Geometry: final body of the model. Coordinates: model frame, mm. Face numbers are marked on the shaded views. A direction names the side the tool comes from. Give positions to 0.01 mm unless a question says otherwise; leave off trailing zeros. Write each loop counter-clockwise with the first axis right and the second up, starting at its lowest first coordinate (ties: lowest second). Pieces come first, ordered by that corner, then holes.
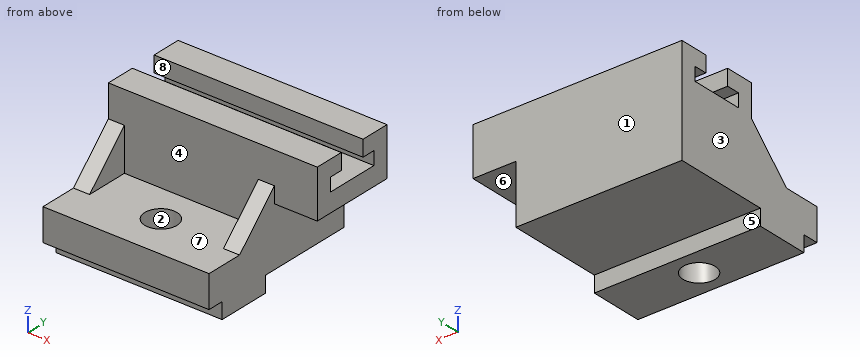
from build123d import *

# Parameters (mm, degrees)
F0_W      = 98.425
F0_H      = 19.05
F1_DEPTH  = 98.425
F2_W      = 98.425
F2_H      = 31.75
F3_DEPTH  = 9.525
F5_DEPTH  = 58.928
F6_W      = 98.425
F6_H      = 50.8
F7_DEPTH  = 44.45
F8_W      = 98.425
F8_H      = 15.875
F9_DEPTH  = 17.4625
F10_W     = 7.9375
F10_H     = 7.9375
F11_DEPTH = 104.394
F13_DEPTH = 25.4
F14_W     = 9.525
F14_H     = 25.4
F15_DEPTH = 31.242
F17_DEPTH = 25.4
F19_DEPTH = 39.878
F21_DEPTH = 25.4


with BuildPart() as f1:
    # F0 (on Front) → F1 (new body)
    with BuildSketch(Plane.XZ):
        with Locations((16.241223073, -7.6058536083)):
            Rectangle(F0_W, F0_H)
    extrude(amount=F1_DEPTH)

    # F2 (on face) → F3 (join)
    with BuildSketch(Plane(origin=(0, 0, -17.1308536083), x_dir=(1, 0, 0), z_dir=(0, 0, -1))):
        with Locations((16.241223073, 73.025)):
            Rectangle(F2_W, F2_H)
    extrude(amount=F3_DEPTH)

    # F4 (on face) → F5 (cut)
    with BuildSketch(Plane.XY.offset(1.9191463917)):
        with BuildLine():
            ThreePointArc((16.241223073, -82.55), (22.9764151638, -79.7601920908), (25.766223073, -73.025))
            ThreePointArc((25.766223073, -73.025), (9.5060309822, -66.2898079092), (16.241223073, -82.55))
        make_face()
    extrude(amount=-F5_DEPTH, mode=Mode.SUBTRACT)

    # F6 (on face) → F7 (join)
    with BuildSketch(Plane.XY.offset(1.9191463917)):
        with Locations((16.241223073, -25.4)):
            Rectangle(F6_W, F6_H)
    extrude(amount=F7_DEPTH)

    # F8 (on face) → F9 (cut)
    with BuildSketch(Plane.XY.offset(46.3691463917)):
        with Locations((16.241223073, -25.4)):
            Rectangle(F8_W, F8_H)
    extrude(amount=-F9_DEPTH, mode=Mode.SUBTRACT)

    # F10 (on face) → F11 (cut)
    with BuildSketch(Plane(origin=(-32.971276927, 0, 0), x_dir=(0, -1, 0), z_dir=(-1, 0, 0))):
        with Locations((13.49375, 32.8753963917)):
            Rectangle(F10_W, F10_H)
        with Locations((37.30625, 32.8753963917)):
            Rectangle(F10_W, F10_H)
    extrude(amount=-F11_DEPTH, mode=Mode.SUBTRACT)

    # F12 (on face) → F13 (join)
    with BuildSketch(Plane.YZ.offset(65.453723073)):
        Polygon((-33.3375, 46.3691463917), (-50.8, 46.3691463917), (-50.8, 17.7941463917), (0, 17.7941463917), (0, 46.3691463917), (-17.4625, 46.3691463917), (-17.4625, 36.8441463917), (-9.525, 36.8441463917), (-9.525, 28.9066463917), (-41.275, 28.9066463917), (-41.275, 36.8441463917), (-33.3375, 36.8441463917), align=None)
    extrude(amount=F13_DEPTH)

    # F14 (on face) → F15 (join)
    with BuildSketch(Plane.XZ.offset(50.8)):
        with Locations((-28.208776927, 14.6191463917)):
            Rectangle(F14_W, F14_H)
    extrude(amount=F15_DEPTH)

    # F16 (on face) → F17 (cut)
    with BuildSketch(Plane.YZ.offset(-23.446276927)):
        Polygon((-76.2, 1.9191463917), (-50.8, 27.3191463917), (-82.042, 27.3191463917), (-82.042, 1.9191463917), align=None)
    extrude(amount=-F17_DEPTH, mode=Mode.SUBTRACT)

    # F18 (on face) → F19 (join)
    with BuildSketch(Plane.XZ.offset(50.8)):
        Polygon((55.928723073, 1.9191463917), (65.453723073, 1.9191463917), (65.453723073, 17.7941463917), (65.453723073, 27.3191463917), (55.928723073, 27.3191463917), align=None)
    extrude(amount=F19_DEPTH)

    # F20 (on face) → F21 (cut)
    with BuildSketch(Plane(origin=(55.928723073, 0, 0), x_dir=(0, -1, 0), z_dir=(-1, 0, 0))):
        Polygon((90.678, 27.3191463917), (50.8, 27.3191463917), (76.2, 1.9191463917), (90.678, 1.9191463917), align=None)
    extrude(amount=-F21_DEPTH, mode=Mode.SUBTRACT)


solid = f1.part
Q1. Section D-D on y = -43.5. Output: boundary loops of the cut face in (x, z), plus the area to 3 significant figures.
Filled sheet:
outline: (-32.97, -17.13) - (65.45, -17.13) - (65.45, 17.79) - (90.85, 17.79) - (90.85, 46.37) - (-32.97, 46.37) - close
area: 6,980 mm2
Q2. Pull-direction query (X, two-part tool) for the marked faces 1, 2, 3 and 4; classes: released by +X, released by -X, zero draft, split by the parting line, or undercut.
Filled sheet:
face 1: zero draft
face 2: undercut
face 3: released by -X
face 4: undercut
Q3. Section C-C on y = -80.5. Output: boundary loops of the cut face in (x, z), plus the area to 3 significant figures.
Filled sheet:
outline: (-32.97, -26.66) - (10.34, -26.66) - (10.34, 1.92) - (-32.97, 1.92) - close; (22.14, -26.66) - (65.45, -26.66) - (65.45, 1.92) - (22.14, 1.92) - close
area: 2,480 mm2
Q4. Access query for the marked faces 5, 6, 7 and 8. Directions: +Z, -Z, +X, -X, +Y, -Y. A direction counts if a zero-diameter tool reaches every point of the face in a straight line with its end or side. Return the directions, or none.
Filled sheet:
face 5: -Z, +X, -X, +Y
face 6: -Z, +X, +Y, -Y
face 7: +Z, -Y
face 8: +Z, +X, -X
Q5. Section A-A on z = 31.5. Output: boundary loops of the cut face in (x, y) (3 decimals), plus the area to 3 significant figures.
Filled sheet:
outline: (-32.971, -50.8) - (90.854, -50.8) - (90.854, -41.275) - (-32.971, -41.275) - close; (-32.971, -9.525) - (90.854, -9.525) - (90.854, 0) - (-32.971, 0) - close
area: 2,360 mm2
Q6. Ray query, line 1 along Z through (x, y) = (15.5, -12); line 2 along Y through (x, z) = (-19, 31) (3 decimals); line 3 along X through (y, z) = (-65.5, 9). Return the intervals inside material, ascending.
Filled sheet:
line 1: z = -17.13 to 28.91, 36.84 to 46.37
line 2: y = -50.8 to -41.275, -9.525 to 0
line 3: x = -32.97 to -23.45, 55.93 to 65.45
Q7. Pin query (flat end, axial travel): P1, Ø17, axis at x = 34.5, y = -26, coming from the -Z side; P2, Ø6, axis at y = -20.5, z = 2, coming from the +X side; P3, Ø7.5, axis at x = 76.5, y = -26.5, coming from the -Z side; P4, Ø3, axis at x = 59, z = 43, coming from the +Y side. Return the tip coordinate at first contact, or that it passes through.
Filled sheet:
P1: stops at z = -17.13
P2: stops at x = 65.45
P3: stops at z = 17.79
P4: stops at y = 0
